Geometry check sheet. Reference: the model listing, model coordinates, mm. A direction names the side the tool comes from. Coordinates: 2 decimals unless noted, no trailing zeros. Loops run counter-clockwise (first coordinate to the right, second up) from the corner with the lowest first, then second, coordinate; pieces in that order, holes last.
from build123d import *

# Parameters (mm, degrees)
F1_DEPTH = 3.5
F2_R     = 1


with BuildPart() as f1:
    # F0 (on Top) → F1 (new body, symmetric)
    with BuildSketch(Plane.XY):
        Polygon((25.980762, -15), (0, 30), (-25.980762, -15), align=None)
        with BuildLine():
            Line((-5.5, 9.526279), (0, 24))
            Line((0, 24), (5.5, 9.526279))
            ThreePointArc((5.5, 9.526279), (9.526279, 5.5), (11, 0))
            Line((11, 0), (19.980762, -11.535898))
            Line((19.980762, -11.535898), (5.5, -9.526279))
            ThreePointArc((5.5, -9.526279), (0, -11), (-5.5, -9.526279))
            Line((-5.5, -9.526279), (-19.980762, -11.535898))
            Line((-19.980762, -11.535898), (-11, 0))
            ThreePointArc((-11, 0), (-9.526279, 5.5), (-5.5, 9.526279))
        make_face(mode=Mode.SUBTRACT)
    extrude(amount=F1_DEPTH, both=True)

    # F2
    f2_edges = [f1.edges().sort_by_distance(p)[0] for p in [
        (0, -15, -3.5),
        (25.980762, -15, 0),
        (0, -15, 3.5),
        (-25.980762, -15, 0),
        (12.990381, 7.5, 3.5),
        (-12.990381, 7.5, 3.5),
        (-2.75, 16.76314, 3.5),
        (2.75, 16.76314, 3.5),
        (9.526279, 5.5, 3.5),
        (15.490381, -5.767949, 3.5),
        (12.740381, -10.531089, 3.5),
        (0, -11, 3.5),
        (-12.740381, -10.531089, 3.5),
        (-15.490381, -5.767949, 3.5),
        (-9.526279, 5.5, 3.5),
        (-19.980762, -11.535898, 0),
        (-15.490381, -5.767949, -3.5),
        (-11, 0, 0),
        (-2.75, 16.76314, -3.5),
        (0, 24, 0),
        (-5.5, 9.526279, 0),
        (2.75, 16.76314, -3.5),
        (5.5, 9.526279, 0),
        (9.526279, 5.5, -3.5),
        (11, 0, 0),
        (15.490381, -5.767949, -3.5),
        (19.980762, -11.535898, 0),
        (12.990381, 7.5, -3.5),
        (-12.990381, 7.5, -3.5),
        (12.740381, -10.531089, -3.5),
        (0, -11, -3.5),
        (-12.740381, -10.531089, -3.5),
        (-9.526279, 5.5, -3.5),
        (0, 30, 0),
    ]]
    fillet(f2_edges, radius=F2_R)


solid = f1.part
1) Material ranges on probe 1 along Y at (x, z) = (15.5, 3); probe 2 along X at (y, z) = (17, 2.75); probe 3 along X at (y, z) = (-8, -1.5), recorded low to high.
Data:
probe 1: y = -14.87 to -11.05, -5.56 to 2.89
probe 2: x = -7.47 to -2.69, 2.69 to 7.47
probe 3: x = -21.94 to -17.23, 17.23 to 21.94
2) Mould release check, pull along X, two halves, no side actions. Record for faces 4 (the cylindrical face through (0, 29, 0)), 5 (the cylindrical face through (9.49, 5.56, 0.04)), 6 (the flat face through (-4, -12, 3.5)), 7 (the cylindrical face through (25.12, -14.49, -0.04)): +X half, -X half, draft (parallel to the pull), parting line (faces both ways), or undercut.
Data:
face 4: parting line
face 5: undercut
face 6: draft
face 7: +X half
3) Depth check by flat-ended pin: pin 1 (1.5 mm diameter, centred on y = 6.5, z = 2.5, fed in from -X); pin 2 (1 mm diameter, centred on x = -18.5, z = 2.5, fed in from +Y); pin 3 (10 mm diameter, centred on x = -9, y = -7.5, fed in from -Z); pin 4 (2 mm diameter, centred on y = 10.5, z = -2, fed in from -X). Enter the tip coordinate at first touch or a pass-through.
Data:
pin 1: stops at x = -14
pin 2: stops at y = -1.18
pin 3: stops at z = -3.5
pin 4: stops at x = -11.84
4) Section check A-A on z = -1. Record the cut outline in (x, y), and give its area (3 significant figures).
Data:
outline: (-25.11, -13.5) arc R1 ccw to (-24.25, -15) - (24.25, -15) arc R1 ccw to (25.11, -13.5) - (0.87, 28.5) arc R1 ccw to (-0.87, 28.5) - close; hole (-18.47, -9.59) arc R1 ccw to (-17.54, -11.2) - (-5.5, -9.53) arc R11 ccw to (5.5, -9.53) - (17.54, -11.2) arc R1 ccw to (18.47, -9.59) - (11.21, -0.26) arc R1 cw to (11, 0.32) arc R11 ccw to (5.79, 9.36) arc R1 cw to (5.38, 9.85) - (0.93, 21.54) arc R1 ccw to (-0.93, 21.54) - (-5.38, 9.85) arc R1 cw to (-5.79, 9.36) arc R11 ccw to (-11, 0.32) arc R1 cw to (-11.21, -0.26) - close
area: 595 mm2
5) Access from +Z, -Z, +X, -X, +Y, -Y to the whole of each face (thin tool, end or side, straight path). Record for faces 1 (the cylindrical face through (15.1, -4.8, 3.2)), 2 (the flat face through (3.125, 15.777, 0.035)), 3 (the cylindrical face through (15.1, -4.8, -3.2)).
Data:
face 1: +Z
face 2: +Z, -Z
face 3: -Z
